Geometry check sheet. Reference: the model listing, model coordinates, mm. Face numbers are marked on the shaded views. A direction names the side the tool comes from. Coordinates: 2 decimals unless noted, no trailing zeros. Order: outer loops, then holes, each group sorted by start corner. A loop starts at its lowest first (then second) coordinate and runs counter-clockwise, first axis right, second up. Notation, with made-up numbers: (-11, 49.5) - (43, 49.5) arc R8 ccw to (43, 63.5) - close; hole circle Ø8 at (-32, 7.5). An arc over 180 degrees is marked (long way). Return JSON: item names as keys, results as strings. Group by question number.
Item 1: Gauge pin test, flat end, axial feed: pin 1 (6 mm diameter, centred on x = 23, z = -13.5, fed in from -Y). Record the tip position at first contact, or that the pin passes through.
Item 2: Scan lines: probe 1 along Z at (x, y) = (47.5, 3.75); probe 2 along Y at (x, z) = (26, -8.5). Record each from-to range of solid material in increasing order.
Item 3: Tool access check on the marked faces 1 and 2. Record the directions out of +Z, -Z, +X, -X, +Y, -Y that give a thin tool (end or side, any length) a straight path to the whole face; none if there is none.
Item 4: Section check C-C on z = -5. Enter the section's corners in (x, y).
Item 5: Section check B-B on x = 32. Enter the section's corners in (y, z).
Item 6: Section check A-A on y = 12. Enter the section's corners in (x, z), then the cut area to 3 significant figures.
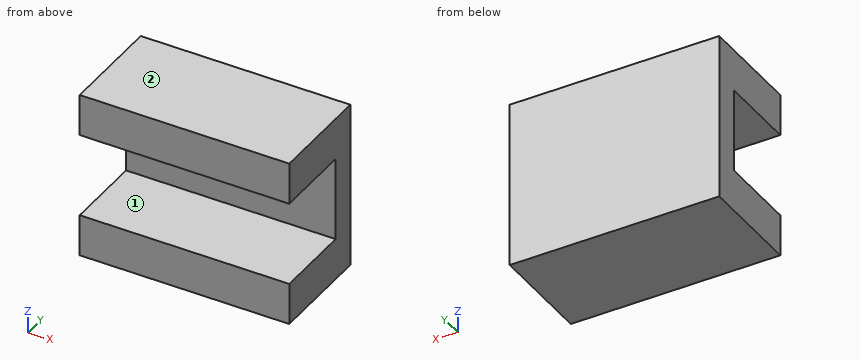
from build123d import *

# Parameters (mm, degrees)
ESBO_O1_W                = 50
ESBO_O1_H                = 25
RESSALTO_EXTRUS_O1_DEPTH = 10
ESBO_O2_W                = 50
ESBO_O2_H                = 20
RESSALTO_EXTRUS_O2_DEPTH = 6
ESBO_O3_W                = 50
ESBO_O3_H                = 25
RESSALTO_EXTRUS_O3_DEPTH = 10


with BuildPart() as part:
    # Esboço1 → Ressalto-extrusão1 (new body)
    with BuildSketch(Plane.XY):
        with Locations((25, 12.5)):
            Rectangle(ESBO_O1_W, ESBO_O1_H)
    extrude(amount=RESSALTO_EXTRUS_O1_DEPTH)

    # Esboço2 → Ressalto-extrusão2 (add)
    with BuildSketch(Plane(origin=(0, 25, 0), x_dir=(1, 0, 0), z_dir=(0, 1, 0))):
        with Locations((25, 10)):
            Rectangle(ESBO_O2_W, ESBO_O2_H)
    extrude(amount=-RESSALTO_EXTRUS_O2_DEPTH)

    # Esboço3 → Ressalto-extrusão3 (add)
    with BuildSketch(Plane(origin=(0, 0, -20), x_dir=(-1, 0, 0), z_dir=(0, 0, -1))):
        with Locations((-25, 12.5)):
            Rectangle(ESBO_O3_W, ESBO_O3_H)
    extrude(amount=RESSALTO_EXTRUS_O3_DEPTH)


solid = part.part
Computed:
{
 "1": {"pin 1": "stops at y = 19"},
 "2": {"probe 1": "z = -30 to -20, 0 to 10", "probe 2": "y = 19 to 25"},
 "3": {"face 1": "+X, -X, -Y", "face 2": "+Z, +X, -X, +Y, -Y"},
 "4": {"outline": "(0, 19) - (50, 19) - (50, 25) - (0, 25) - close"},
 "5": {"outline": "(0, -30) - (25, -30) - (25, 10) - (0, 10) - (0, 0) - (19, 0) - (19, -20) - (0, -20) - close"},
 "6": {"outline": "(0, -30) - (50, -30) - (50, -20) - (0, -20) - close; (0, 0) - (50, 0) - (50, 10) - (0, 10) - close", "area": "1,000 mm²"}
}
